Work out the finished part from the listing and answer in its coordinate system (mm). A direction names the side the tool comes from. Coordinates: 2 decimals unless noted, no trailing zeros. Write each loop counter-clockwise with the first axis right and the second up, starting at its lowest first coordinate (ties: lowest second). Pieces come first, ordered by that corner, then holes. Notation, with made-up numbers: (-39.5, -0.75) - (-22.5, -0.75) arc R19 ccw to (-22.5, 36.25) - close; hole circle Ø11 at (-11, 78). An arc over 180 degrees is marked (long way). Use a Markdown table: item, result. Add a question column.
(1) For a pull along Y with two mould halves and no side action, classify faces 4 (the face through (5.028, -22.677, -33.861)), 5 (the face through (-2.47, -8.43, 4.38)), 6 (the face through (2.493, -10.648, 13.887)), 7 (the face through (2, -4, -4)) as released by +Y, released by -Y, zero draft, split by the parting line, or undercut.
(2) The part is cut by section D-D, the plane z = -39. Give the vertices of the cut face in (x, y).
(3) The part is cut by section B-B, the plane x = -2. Give the vertices of the cut face in (y, z).
(4) Given pin 1 Ø4 at (x, y) = (-2.5, 8) entering from -Z; pin 2 Ø2 at (y, z) = (6.75, -71.69) entering from +X; pin 3 Ø8 at (y, z) = (16, -37.5) entering from -X; pin 4 Ø1.5 at (x, y) = (1.5, -2) entering from -Z, each flat-ended and moving along its own axis, determine where each tip first touches the part or whether it passes through.
(5) The part is cut by section C-C, the plane y = -22.5. Give the vertices of the cut face in (x, z).
(6) A tool of negligible diameter and unlimited length cuts with its end or side. For faces 1 (the face through (5, -8.4, -57.8)), 2 (the face through (-2.535, -5.536, -0.325)), 3 (the face through (3.451, -12.011, 18.494)), from which of +Z, -Z, +X, -X, +Y, -Y can it reach the whole face along a straight path? Write none if from no direction.
(7) The part is cut by section A-A, the plane y = 13.5. Give the vertices of the cut face in (x, z), then the cut area to 3 significant figures.
(8) Find the intervals of material crossed by line 1 (Y direction, x = -1.2, z = 0); line 2 (Y direction, x = 5.5, z = 0); line 3 (Y direction, x = -3.85, z = 0), in increasing order. Write a range as from..to.
from build123d import *

# Parameters (mm, degrees)
SKETCH_3_R                   = 27.5
EXTRUDE_1_DEPTH              = 2
SKETCH_4_R                   = 27.5
SKETCH_4_R_2                 = 17.5
EXTRUDE_2_DEPTH              = 1
SKETCH_5_R                   = 27.5
SKETCH_5_R_2                 = 18.5
EXTRUDE_3_DEPTH              = 7
SKETCH_6_R                   = 27.5
SKETCH_6_R_2                 = 17.5
EXTRUDE_4_DEPTH              = 2
EXTRUDE_5_DEPTH              = 9
SKETCH_11_R                  = 8.5
CUT_EXTRUDE_3_DEPTH          = 111
SKETCH_12_R                  = 9.5
CUT_EXTRUDE_4_DEPTH          = 2.5
SKETCH_13_R                  = 9.5
EXTRUDE_6_DEPTH              = 5
SKETCH_17_W                  = 17.714059585
SKETCH_17_H                  = 64.604217311
CUT_EXTRUDE_5_DEPTH          = 1111
HOLE_WIZARD_M3_1_D           = 2.5
PATTERN_CIRCULAR_2_COUNT     = 6
HOLE_WIZARD_M3_2_D           = 2.5
PATTERN_CIRCULAR_3_COUNT     = 6
SKETCH_26_R                  = 27.5
SKETCH_26_R_2                = 25
CUT_EXTRUDE_6_DEPTH          = 1
FILLET_1_R                   = 0.1
PATTERN_CIRCULAR_4_COUNT     = 3
HOLE_WIZARD_M5_1_D           = 5.3
HOLE_WIZARD_M5_1_CBORE_D     = 10
HOLE_WIZARD_M5_1_CBORE_DEPTH = 5.4


with BuildPart() as part:
    # 스케치3 → 보스-돌출1 (new body)
    with BuildSketch(Plane(origin=(0, 0, 0), x_dir=(0, 0, -1), z_dir=(1, 0, 0))):
        Circle(SKETCH_3_R)
    extrude(amount=EXTRUDE_1_DEPTH)

    # 스케치4 → 보스-돌출2 (add)
    with BuildSketch(Plane(origin=(2, 0, 0), x_dir=(0, 0, -1), z_dir=(1, 0, 0))):
        Circle(SKETCH_4_R)
        Circle(SKETCH_4_R_2, mode=Mode.SUBTRACT)
    extrude(amount=EXTRUDE_2_DEPTH)

    # 스케치5 → 보스-돌출3 (add)
    with BuildSketch(Plane(origin=(3, 0, 0), x_dir=(0, 0, -1), z_dir=(1, 0, 0))):
        Circle(SKETCH_5_R)
        Circle(SKETCH_5_R_2, mode=Mode.SUBTRACT)
    extrude(amount=EXTRUDE_3_DEPTH)

    # 스케치6 → 보스-돌출4 (add)
    with BuildSketch(Plane(origin=(10, 0, 0), x_dir=(0, 0, -1), z_dir=(1, 0, 0))):
        Circle(SKETCH_6_R)
        Circle(SKETCH_6_R_2, mode=Mode.SUBTRACT)
    extrude(amount=EXTRUDE_4_DEPTH)

    # 스케치10 → 보스-돌출5 (add)
    with BuildSketch(Plane(origin=(12, 0, 0), x_dir=(0, 0, -1), z_dir=(1, 0, 0))):
        with BuildLine():
            Line((4.125, 27.188864908), (62.775, 18.290690938))
            ThreePointArc((62.775, 18.290690938), (78.5, 0), (62.775, -18.290690938))
            Line((62.775, -18.290690938), (4.125, -27.188864908))
            ThreePointArc((4.125, -27.188864908), (27.5, 0), (4.125, 27.188864908))
        make_face()
    extrude(amount=-EXTRUDE_5_DEPTH)

    # 스케치11 → 컷-돌출3 (cut, symmetric)
    with BuildSketch(Plane(origin=(7.5, 0, 0), x_dir=(0, 0, -1), z_dir=(1, 0, 0))):
        with Locations((60, 0)):
            Circle(SKETCH_11_R)
    extrude(amount=CUT_EXTRUDE_3_DEPTH, both=True, mode=Mode.SUBTRACT)

    # 스케치12 → 컷-돌출4 (cut, symmetric)
    with BuildSketch(Plane(origin=(7.5, 0, 0), x_dir=(0, 0, -1), z_dir=(1, 0, 0))):
        with Locations((60, 0)):
            Circle(SKETCH_12_R)
    extrude(amount=CUT_EXTRUDE_4_DEPTH, both=True, mode=Mode.SUBTRACT)

    # 스케치13 → 보스-돌출6 (add)
    with BuildSketch(Plane.ZY):
        Circle(SKETCH_13_R)
    extrude(amount=EXTRUDE_6_DEPTH)

    # 스케치17 → 컷-돌출5 (cut, symmetric)
    with BuildSketch(Plane.XY):
        with Locations((15.857029793, -1.852450676)):
            Rectangle(SKETCH_17_W, SKETCH_17_H)
    extrude(amount=CUT_EXTRUDE_5_DEPTH, both=True, mode=Mode.SUBTRACT)

    # Hole Wizard M3 _ _ _ _1 (through all)
    with Locations(Plane(origin=(7, 0, 0), x_dir=(0, 0, -1), z_dir=(1, 0, 0))):
        with Locations((0, 22.5)):
            hole_wizard_m3_1 = Hole(HOLE_WIZARD_M3_1_D / 2)

    # 원형 패턴2: Hole Wizard M3 _ _ _ _1 ×6 about axis
    pattern_circular_2_axis = Axis((0, 0, 0), (1, 0, 0))
    for i in range(1, PATTERN_CIRCULAR_2_COUNT):
        add(hole_wizard_m3_1.rotate(pattern_circular_2_axis, i * 360 / PATTERN_CIRCULAR_2_COUNT), mode=Mode.SUBTRACT)

    # M3 탭을 위한 탭 드릴2 (through all)
    with Locations(Plane(origin=(7, 0, 0), x_dir=(0, 0, -1), z_dir=(1, 0, 0))):
        with Locations((60, 13.5)):
            hole_wizard_m3_2 = Hole(HOLE_WIZARD_M3_2_D / 2)

    # 원형 패턴3: M3 탭을 위한 탭 드릴2 ×6 about axis
    pattern_circular_3_axis = Axis((0, 0, -60), (1, 0, 0))
    for i in range(1, PATTERN_CIRCULAR_3_COUNT):
        add(hole_wizard_m3_2.rotate(pattern_circular_3_axis, i * 360 / PATTERN_CIRCULAR_3_COUNT), mode=Mode.SUBTRACT)

    # 스케치26 → 컷-돌출6 (cut)
    with BuildSketch(Plane.ZY):
        Circle(SKETCH_26_R)
        Circle(SKETCH_26_R_2, mode=Mode.SUBTRACT)
    extrude(amount=-CUT_EXTRUDE_6_DEPTH, mode=Mode.SUBTRACT)

    # 필렛1
    fillet_1_edges = [part.edges().sort_by_distance(p)[0] for p in [
        (0, 0, -9.5),
        (-5, 0, -9.5),
    ]]
    fillet(fillet_1_edges, radius=FILLET_1_R)

    # 스케치29 → Ø3.0mm 맞춤핀 구멍1 (revolve, cut)
    with BuildSketch(Plane(origin=(-5, -7, 0), x_dir=(0, 0, 1), z_dir=(0, 1, 0))):
        Polygon((0, 0), (0, 5.901290929), (1.5, 5), (1.5, 0), align=None)
    f_3_0mm_1 = revolve(axis=Axis((-11.35, -7, 0), (1, 0, 0)), mode=Mode.SUBTRACT)

    # 원형 패턴4: Ø3.0mm 맞춤핀 구멍1 ×3 about axis
    pattern_circular_4_axis = Axis((0, 0, 0), (1, 0, 0))
    for i in range(1, PATTERN_CIRCULAR_4_COUNT):
        add(f_3_0mm_1.rotate(pattern_circular_4_axis, i * 360 / PATTERN_CIRCULAR_4_COUNT), mode=Mode.SUBTRACT)

    # M5 육각 소켓 머리 캡 나사용 카운터보어1 (through all)
    with Locations(Plane(origin=(2, 0, 0), x_dir=(0, 0, -1), z_dir=(1, 0, 0))):
        with Locations((0, 0)):
            CounterBoreHole(HOLE_WIZARD_M5_1_D / 2, HOLE_WIZARD_M5_1_CBORE_D / 2, HOLE_WIZARD_M5_1_CBORE_DEPTH)


solid = part.part
Model answer:
| question | item | result |
|---|---|---|
| 1 | face 4 | released by -Y |
| 1 | face 5 | split by the parting line |
| 1 | face 6 | undercut |
| 1 | face 7 | undercut |
| 2 | outline | (3, -21.9) - (7, -21.9) - (7, 21.9) - (3, 21.9) - close |
| 3 | outline | circle Ø19 at (0, 0); hole circle Ø3 at (-7, 0); hole circle Ø10 at (0, 0); hole circle Ø3 at (3.5, -6.06); hole circle Ø3 at (3.5, 6.06) |
| 4 | pin 1 | z = -7.37 |
| 4 | pin 2 | through |
| 4 | pin 3 | x = 3 |
| 4 | pin 4 | z = -27.47 |
| 5 | outline | (0, -10.9) - (1, -10.9) - (1, -15.81) - (3, -15.81) - (3, -35.03) - (7, -35.03) - (7, -1.25) - (0, -1.25) - close; (0, 1.25) - (7, 1.25) - (7, 15.81) - (1, 15.81) - (1, 10.9) - (0, 10.9) - close |
| 6 | face 1 | +X |
| 6 | face 2 | -X |
| 6 | face 3 | +X, -X |
| 7 | outline | (0, -21.04) - (1, -21.04) - (1, -23.96) - (3, -23.96) - (3, -58.75) - (7, -58.75) - (7, -12.65) - (3, -12.65) - (3, -11.14) - (2, -11.14) - (2, 11.14) - (3, 11.14) - (3, 12.65) - (7, 12.65) - (7, 23.96) - (1, 23.96) - (1, 21.04) - (0, 21.04) - close; (3, -72.65) - (7, -72.65) - (7, -61.25) - (3, -61.25) - close |
| 7 | area | 391 mm^2 |
| 8 | line 1 | -9.5..-8.5, -5.5..-5, 5..9.5 |
| 8 | line 2 | -27.5..-23.75, -21.25..-18.5, 18.5..21.25, 23.75..27.5 |
| 8 | line 3 | -9.5..-8.5, -5.5..-2.65, 2.65..9.5 |
